Source: CAD feature listing. Evaluate the final solid. Frame: model axes, mm. Face numbers are marked on the shaded views. A direction names the side the tool comes from. Coordinates: 2 decimals unless noted, no trailing zeros. Order: outer loops, then holes, each group sorted by start corner. A loop starts at its lowest first (then second) coordinate and runs counter-clockwise, first axis right, second up. Notation, with made-up numbers: (-8.75, 21.5) - (20.25, 21.5) arc R7 ccw to (20.25, 29.5) - close; hole circle Ø1 at (52, -17). An arc over 180 degrees is marked (long way). One line per question, with ' | ' between items. Start each with the question number.
(1) Line query: line 1 along Z through (x, y) = (0, 4.1); line 2 along Z through (x, y) = (-35.5, 5.75); line 3 along X through (y, z) = (1.5, 13) (3 decimals). Output: solid intervals per line, ascending.
(2) Section C-C (x = -1). Return the cut outline in (y, z).
(3) Section B-B (y = 7). Return the cut outline in (x, z) (3 decimals).
(4) Access query for the marked faces 1, 2 and 3. Directions: +Z, -Z, +X, -X, +Y, -Y. A direction counts if a zero-diameter tool reaches every point of the face in a straight line with its end or side. Return the directions, or none.
(5) Draft query along X for the marked faces 4, 5 and 6. Return one class per face: +X half, -X half, draft (parallel to the pull), parting line (faces both ways), or undercut.
(6) Contact query for flat-ended pins moving along their axis: P1, Ø4.5, axis at x = 0, z = 13.47, coming from the +Y side; P2, Ø7, axis at x = -31, z = -13, coming from the -Y side. Output: stop coordinate, or through.
(7) Section D-D (z = 10.5). Return the cut outline in (x, y) (3 decimals).
(8) Section A-A (x = -23.5). Return the cut outline in (y, z), then the cut area to 3 significant figures.
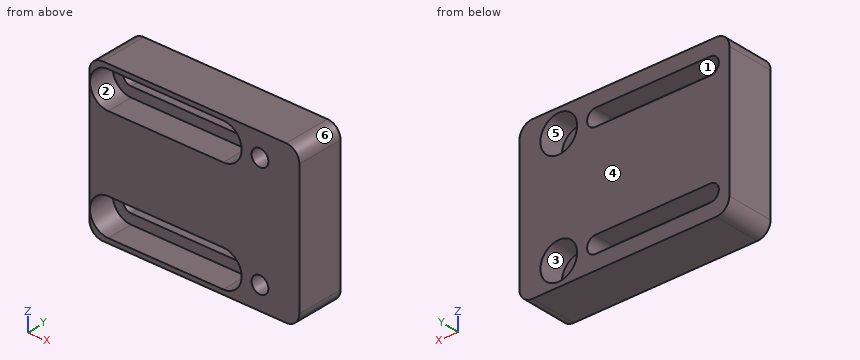
Autodesk Inventor part; units mm, degrees
ref_plane "XZ Plane" through (0, 0, 0) normal (0, 1, 0) x (-1, 0, 0)
ref_plane "XY Plane" through (0, 0, 0) normal (0, 0, 1) x (1, 0, 0)
sketch "Sketch1" plane through (0, 0, 0) normal (0, 1, 0) x (-1, 0, 0)
  line L0 (-9.525, 19.05) -> (41.275, 19.05)
  line L1 (41.275, 19.05) -> (41.275, -19.05)
  line L2 (41.275, -19.05) -> (-9.525, -19.05)
  line L3 (-9.525, -19.05) -> (-9.525, 19.05)
  point P0 (0, 0)
  dimension "d0" = 50.8
  dimension "d1" = 38.1
  dimension "d3" = 9.525
  dimension "d4" = 19.05
extrude "Extrusion1" add sketch "Sketch1" along normal blind 11.43
sketch "Sketch2" plane through (0, 11.43, 0) normal (0, 1, 0) x (1, 0, 0)
  line L0 (9.525, -19.05) -> (9.525, 19.05)
  point P0 (0, 0)
  point P1 (0, -13.4747)
  point P2 (0, 13.4747)
  dimension "d7" = 26.9494
  dimension "d9" = 9.525
  dimension "d10" = 9.525
  dimension "d11" = 13.4747
hole "Hole1" at (0, 11.43, 13.4747) at (0, 11.43, -13.4747) direction (0, -1, 0) diameter 4.064 end through all counterbore diameter 8.89 counterbore depth 5.9436
sketch "Sketch3" plane through (0, 0, 0) normal (0, -1, 0) x (1, 0, 0)
  circle A0 centre (0, -13.4747) radius 2.032
  circle A1 centre (0, 13.4747) radius 2.032
  line L0 (-41.275, -19.05) -> (-41.275, 19.05)
  line L1 (-36.703, -13.4747) -> (-8.89, -13.4747) construction
  line L2 (-36.703, -15.5067) -> (-8.89, -15.5067)
  line L3 (-8.89, -11.4427) -> (-36.703, -11.4427)
  arc A2 (-36.703, -11.4427) -> (-36.703, -15.5067) centre (-36.703, -13.4747) ccw
  arc A3 (-8.89, -15.5067) -> (-8.89, -11.4427) centre (-8.89, -13.4747) ccw
  line L4 (-36.703, 13.4747) -> (-8.89, 13.4747) construction
  line L5 (-36.703, 11.4427) -> (-8.89, 11.4427)
  line L6 (-8.89, 15.5067) -> (-36.703, 15.5067)
  arc A4 (-36.703, 15.5067) -> (-36.703, 11.4427) centre (-36.703, 13.4747) ccw
  arc A5 (-8.89, 11.4427) -> (-8.89, 15.5067) centre (-8.89, 13.4747) ccw
  point P0 (0, 0)
  point P1 (-22.7965, -13.4747)
  point P2 (-22.7965, 13.4747)
  dimension "d19" = 26.9494
  dimension "d20" = 13.4747
  dimension "d21" = 8.89
  dimension "d22" = 8.89
  dimension "d23" = 4.572
  dimension "d24" = 4.572
  dimension "d25" = 4.064
  dimension "d26" = 4.064
extrude "Extrusion2" cut sketch "Sketch3" against normal through all contours A2 L3 A3 L2 | A4 L6 A5 L5
sketch "Sketch4" plane through (0, 0, 0) normal (0, -1, 0) x (1, 0, 0)
  arc A0 (-36.703, 15.5067) -> (-36.703, 11.4427) centre (-36.703, 13.4747) ccw
  arc A1 (-8.89, 11.4427) -> (-8.89, 15.5067) centre (-8.89, 13.4747) ccw
  line L0 (-36.703, 13.4747) -> (-8.89, 13.4747) construction
  line L1 (-36.703, 9.0297) -> (-8.89, 9.0297)
  line L2 (-8.89, 17.9197) -> (-36.703, 17.9197)
  arc A2 (-36.703, 17.9197) -> (-36.703, 9.0297) centre (-36.703, 13.4747) ccw
  arc A3 (-8.89, 9.0297) -> (-8.89, 17.9197) centre (-8.89, 13.4747) ccw
  arc A4 (-8.89, -15.5067) -> (-8.89, -11.4427) centre (-8.89, -13.4747) ccw
  arc A5 (-36.703, -11.4427) -> (-36.703, -15.5067) centre (-36.703, -13.4747) ccw
  line L3 (-8.89, -13.4747) -> (-36.703, -13.4747) construction
  line L4 (-8.89, -9.0297) -> (-36.703, -9.0297)
  line L5 (-36.703, -17.9197) -> (-8.89, -17.9197)
  arc A6 (-8.89, -17.9197) -> (-8.89, -9.0297) centre (-8.89, -13.4747) ccw
  arc A7 (-36.703, -9.0297) -> (-36.703, -17.9197) centre (-36.703, -13.4747) ccw
  point P0 (0, 0)
  point P1 (-22.7965, 13.4747)
  point P2 (-22.7965, -13.4747)
  dimension "d29" = 8.89
  dimension "d30" = 8.89
extrude "Extrusion3" cut sketch "Sketch4" against normal blind 6.35
fillet "Fillet1" radius 3.175 4 edges at (9.525, 5.715, 19.05) (9.525, 5.715, -19.05) (-41.275, 5.715, 19.05) (-41.275, 5.715, -19.05)
equation "\"d22\" = d21"
equation "\"d24\" = d23"
equation "\"d26\" = d25"
equation "\"d30\" = d29"
properties part number "intake wheel only to xrail"
Response values:
1) line 1: z = -19.05 to -15.51, -11.44 to 11.44, 15.51 to 19.05 | line 2: z = -19.05 to -17.92, -9.03 to 9.03, 17.92 to 19.05 | line 3: x = -41.275 to -41.123, -4.47 to -1.976, 1.976 to 9.525
2) outline: (0, -19.05) - (11.43, -19.05) - (11.43, -17.81) - (5.49, -17.81) - (5.49, -15.24) - (0, -15.24) - close; (0, -11.71) - (5.49, -11.71) - (5.49, -9.14) - (11.43, -9.14) - (11.43, 9.14) - (5.49, 9.14) - (5.49, 11.71) - (0, 11.71) - close; (0, 15.24) - (5.49, 15.24) - (5.49, 17.81) - (11.43, 17.81) - (11.43, 19.05) - (0, 19.05) - close
3) outline: (-41.275, -15.875) arc R3.175 ccw to (-38.1, -19.05) - (6.35, -19.05) arc R3.175 ccw to (9.525, -15.875) - (9.525, 15.875) arc R3.175 ccw to (6.35, 19.05) - (-38.1, 19.05) arc R3.175 ccw to (-41.275, 15.875) - close; hole (-36.703, -15.507) - (-8.89, -15.507) arc R2.032 ccw to (-8.89, -11.443) - (-36.703, -11.443) arc R2.032 ccw to start; hole (-36.703, 11.443) - (-8.89, 11.443) arc R2.032 ccw to (-8.89, 15.507) - (-36.703, 15.507) arc R2.032 ccw to start; hole circle Ø8.89 at (0, -13.475); hole circle Ø8.89 at (0, 13.475)
4) face 1: +Y, -Y | face 2: -Y | face 3: +Y
5) face 4: draft | face 5: undercut | face 6: +X half
6) P1: stops at y = 5.49 | P2: stops at y = 6.35
7) outline: (-41.275, 0) - (-40.006, 0) - (-40.006, 6.35) - (-5.587, 6.35) - (-5.587, 0) - (9.525, 0) - (9.525, 11.43) - (3.303, 11.43) - (3.303, 5.486) - (-3.303, 5.486) - (-3.303, 11.43) - (-41.275, 11.43) - close
8) outline: (0, -19.05) - (11.43, -19.05) - (11.43, -15.51) - (6.35, -15.51) - (6.35, -17.92) - (0, -17.92) - close; (0, -9.03) - (6.35, -9.03) - (6.35, -11.44) - (11.43, -11.44) - (11.43, 11.44) - (6.35, 11.44) - (6.35, 9.03) - (0, 9.03) - close; (0, 17.92) - (6.35, 17.92) - (6.35, 15.51) - (11.43, 15.51) - (11.43, 19.05) - (0, 19.05) - close | area: 281 mm²
